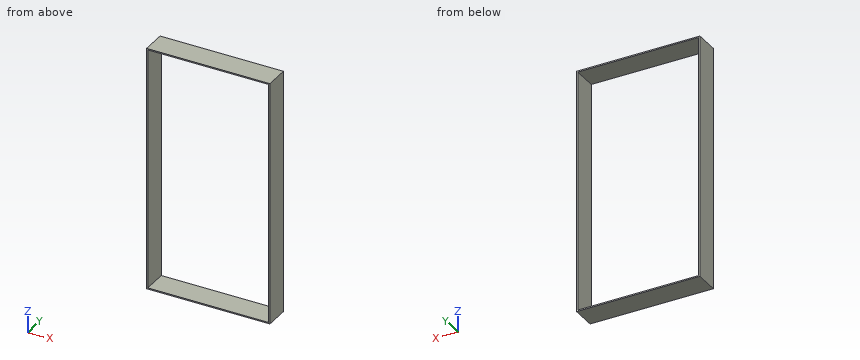
Autodesk Inventor part; units mm, degrees
ref_plane "YZ Plane" through (0, 0, 0) normal (1, 0, 0) x (0, 1, 0)
ref_plane "XZ Plane" through (0, 0, 0) normal (0, 1, 0) x (-1, 0, 0)
ref_plane "XY Plane" through (0, 0, 0) normal (0, 0, 1) x (1, 0, 0)
sketch "Sketch2" plane through (0, 0, 0) normal (0, 1, 0) x (-1, 0, 0)
  line L0 (0, 0) -> (-20, 0)
  line L1 (0, 0) -> (100, 0)
  line L2 (100, 0) -> (100, 200)
  line L3 (100, 200) -> (0, 200)
  line L4 (0, 200) -> (0, 0)
  line L5 (101, 201) -> (-1, 201)
  line L6 (-1, 201) -> (-1, -1)
  line L7 (-1, -1) -> (101, -1)
  line L8 (101, -1) -> (101, 201)
  dimension "d8" = 100
  dimension "d9" = 200
  dimension "d10" = 1
  dimension "d11" = 1
  dimension "d12" = 1
  dimension "d13" = 1
extrude "Extrusion2" add sketch "Sketch2" along normal blind 20
equation "\"d8\" = inner_width"
equation "\"d9\" = height"
equation "\"d10\" = wall_thicknes"
equation "\"d11\" = wall_thicknes"
equation "\"d12\" = wall_thicknes"
equation "\"d13\" = wall_thicknes"
properties part number "vib_bed_full_xz"
Input: part model. Units: mm. Frame: model coordinates. Give positions to 0.01 mm unless a question says otherwise; leave off trailing zeros. Write each loop counter-clockwise with the first axis right and the second up, starting at its lowest first coordinate (ties: lowest second). Pieces come first, ordered by that corner, then holes. Notation, with made-up numbers: (-14, 72.5) - (28, 72.5) arc R21 cw to (28, 106.5) - close; hole circle Ø10 at (36, -14). An arc over 180 degrees is marked (long way). Write item = value, one per line. Start each with the question number.
1) Cut plane C-C (y = 11.5). Return loops of the section in (x, z), and give its area (3 significant figures).
2) Material intervals for L1, parallel to Z at x = -39, y = 6.5; L2, parallel to X at y = 18.25, z = 42, sorted ascending. Write a range as [from, to].
3) Cut plane B-B (z = 159). Return loops of the section in (x, y), and give its area (3 significant figures).
4) Cut plane A-A (x = -18.5). Return loops of the section in (y, z), and give its area (3 significant figures).
Answers follow:
q1.outline = (-101, -1) - (1, -1) - (1, 201) - (-101, 201) - close; hole (-100, 0) - (0, 0) - (0, 200) - (-100, 200) - close
q1.area = 604 mm^2
q2.L1 = [-1, 0], [200, 201]
q2.L2 = [-101, -100], [0, 1]
q3.outline = (-101, 0) - (-100, 0) - (-100, 20) - (-101, 20) - close; (0, 0) - (1, 0) - (1, 20) - (0, 20) - close
q3.area = 40.0 mm^2
q4.outline = (0, -1) - (20, -1) - (20, 0) - (0, 0) - close; (0, 200) - (20, 200) - (20, 201) - (0, 201) - close
q4.area = 40.0 mm^2
